from build123d import *

# Parameters (mm, degrees)
BOSS_EXTRUDE1_DEPTH = 40


with BuildPart() as part:
    # Sketch1 → Boss-Extrude1 (new body)
    with BuildSketch(Plane.XY):
        with BuildLine():
            Line((0, 0), (55, 0))
            Line((55, 0), (55, -43))
            ThreePointArc((55, -43), (85.882739779, -81.947086747), (130.843778303, -60.754536237))
            ThreePointArc((130.843778303, -60.754536237), (127.452045415, -50.70485226), (117.402361439, -54.096585148))
            ThreePointArc((117.402361439, -54.096585148), (89.301712362, -67.341929217), (70, -43))
            Line((70, -43), (70, 12))
            Line((70, 12), (0, 12))
            Line((0, 12), (-15, 6))
            Line((-15, 6), (0, -4))
            Line((0, -4), (0, 0))
        make_face()
    extrude(amount=BOSS_EXTRUDE1_DEPTH)


solid = part.part
The model under review builds one solid part; all positions refer to its coordinate system, in mm. A direction names the side the tool comes from. Give positions to 0.01 mm unless a question says otherwise; leave off trailing zeros. Order: outer loops, then holes, each group sorted by start corner. A loop starts at its lowest first (then second) coordinate and runs counter-clockwise, first axis right, second up. Notation, with made-up numbers: (85.25, 13.25) -> (119.25, 13.25) arc R26 ccw to (119.25, 46.25) -> close; hole circle Ø9 at (-37, 52.5). An arc over 180 degrees is marked (long way). Write item = value, one per line. Start each with the question number.
(1) Take a section at A-A (x = 5). Write out the cut boundary in (y, z), plus the area to 3 significant figures.
(2) For L1, parallel to Y at x = 14.5, z = 33; L2, parallel to X at y = -27, z = 25.5; L3, parallel to Y at x = 108, z = 36.5, list the stretches that pass through material, from the lowest coordinate up. Write a range as from..to.
(3) Take a section at C-C (y = -77). Write out the cut boundary in (x, z), plus the area to 3 significant figures.
(4) For pin 1 Ø1.5 at (y, z) = (-54, 20) entering from -X; pin 2 Ø1 at (y, z) = (-59.5, 25.5) entering from +X; pin 3 Ø2 at (y, z) = (-2, 11.5) entering from +X, all flat-tipped, find the tip position at first contact; note any pin that passes through.
(5) Take a section at B-B (z = 28). Write out the cut boundary in (x, y), plus the area to 3 significant figures.
(6) Tool access review of faces 5 (the flat face through (-7.605, 1.07, 19.72)), 6 (the flat face through (27, 0, 20)): name each direction out of +Z, -Z, +X, -X, +Y, -Y from which nothing blocks a thin tool from reaching the whole face with its end or side.
(7) Draft analysis for pull direction X (two halves, no side actions). For faces 1 (the flat face through (70, -16, 20)), 2 (the flat face through (69, -32, 0)), 3 (the flat face through (0, -2, 20)), 4 (the cylindrical face through (89.76, -67.445, 19.72)), state which applies: +X half, -X half, draft (parallel to the pull), parting line (faces both ways), or undercut.
Returned:
q1.outline = (0, 0) -> (12, 0) -> (12, 40) -> (0, 40) -> close
q1.area = 480 mm²
q2.L1 = 0..12
q2.L2 = 55..70
q2.L3 = -80.83..-64.35
q3.outline = (73.93, 0) -> (116.07, 0) -> (116.07, 40) -> (73.93, 40) -> close
q3.area = 1,690 mm²
q4.pin_1 = 56.34
q4.pin_2 = 131.46
q4.pin_3 = 70
q5.outline = (-15, 6) -> (0, -4) -> (0, 0) -> (55, 0) -> (55, -43) arc R40 ccw to (130.84, -60.75) arc R7.5 ccw to (117.4, -54.1) arc R25 cw to (70, -43) -> (70, 12) -> (0, 12) -> close
q5.area = 3,000 mm²
q6.face_5 = +Z, -Z, -X, -Y
q6.face_6 = +Z, -Z, -Y
q7.face_1 = +X half
q7.face_2 = draft
q7.face_3 = undercut
q7.face_4 = undercut
